The listing builds one solid part. Answer for the finished solid, in the listing's coordinates (mm). Face numbers are marked on the shaded views. A direction names the side the tool comes from. Round coordinates to 2 decimals unless told otherwise and drop trailing zeros. Write each loop counter-clockwise with the first axis right and the second up, starting at its lowest first coordinate (ties: lowest second). Pieces come first, ordered by that corner, then holes.
(1) For the marked faces 4 and 5, determine the directions among +Z, -Z, +X, -X, +Y, -Y from which every point of the face is accessible in a straight line to the end or side of a thin tool.
(2) The mould has two halves that part along Y. Classify the marked faces 1, 2 and 3: +Y half, -Y half, draft (parallel to the pull), parting line (faces both ways), or undercut.
(3) A cutting plane is placed at A-A, the plane z = 7.25. Give the vertices of the cut face in (x, y).
(4) Find the intervals of material crossed by probe 1 along Y at (x, z) = (80, 0.6); probe 2 along X at (y, z) = (37, 9.75); probe 3 along Y at (x, z) = (5, 1.75), in increasing order.
(5) A cutting plane is placed at C-C, the plane x = 31.5. Give the vertices of the cut face in (y, z), and give its area (3 significant figures).
(6) Each of these flat-tipped pins is pushed along its axis until it touches: pin 1 Ø0.8 at (x, z) = (13, 0.5) entering from -Y; pin 2 Ø1.1 at (x, y) = (79.5, 5.5) entering from +Z. Where does it stop, or does it pass through?
(7) A cutting plane is placed at B-B, the plane x = 10. Give the vertices of the cut face in (y, z).
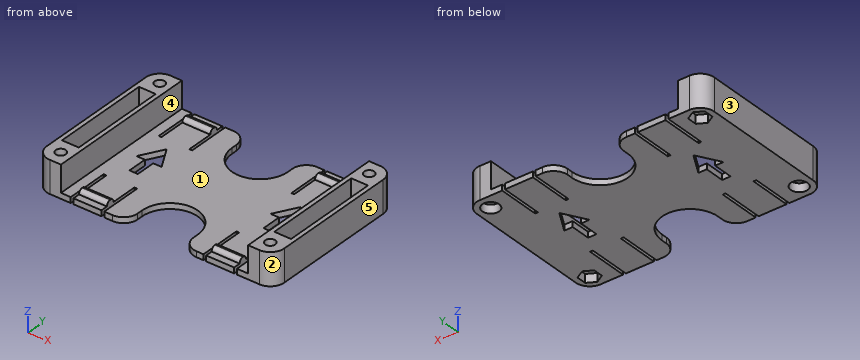
from build123d import *

# Parameters (mm, degrees)
PAD_DEPTH       = 11.5
SKETCH001_W     = 67
SKETCH001_H     = 65
POCKET_DEPTH    = 9.5
SKETCH002_R     = 3
POCKET001_DEPTH = 3
SKETCH003_W     = 6
SKETCH003_H     = 35
POCKET002_DEPTH = 9.5
SKETCH004_R     = 1.8
POCKET003_DEPTH = 8.3
SKETCH006_W     = 1
SKETCH006_H     = 15
POCKET004_DEPTH = 5
SKETCH007_W     = 1
SKETCH007_H     = 15
POCKET005_DEPTH = 5
SKETCH008_W     = 10
SKETCH008_H     = 3
PAD001_DEPTH    = 1.5
FILLET_R        = 1.4
POCKET006_DEPTH = 5


with BuildPart() as part:
    # Sketch → Pad (new body)
    with BuildSketch(Plane.XY):
        with BuildLine():
            ThreePointArc((0, 5), (1.464466, 1.464466), (5, 0))
            Line((5, 0), (27.5, 0))
            ThreePointArc((27.5, 0), (31.035534, 1.464466), (32.5, 5))
            Line((32.5, 5), (32.5, 7))
            ThreePointArc((52.5, 7), (42.5, 17), (32.5, 7))
            Line((52.5, 7), (52.5, 5))
            ThreePointArc((52.5, 5), (53.964466, 1.464466), (57.5, 0))
            Line((57.5, 0), (80, 0))
            ThreePointArc((80, 0), (83.535534, 1.464466), (85, 5))
            Line((85, 50), (85, 5))
            ThreePointArc((85, 50), (83.535534, 53.535534), (80, 55))
            Line((57.5, 55), (80, 55))
            ThreePointArc((57.5, 55), (53.964466, 53.535534), (52.5, 50))
            Line((52.5, 50), (52.5, 48))
            ThreePointArc((32.5, 48), (42.5, 38), (52.5, 48))
            Line((32.5, 50), (32.5, 48))
            ThreePointArc((32.5, 50), (31.035534, 53.535534), (27.5, 55))
            Line((5, 55), (27.5, 55))
            ThreePointArc((5, 55), (1.464466, 53.535534), (0, 50))
            Line((0, 5), (0, 50))
        make_face()
    extrude(amount=PAD_DEPTH)

    # Sketch001 → Pocket (cut)
    with BuildSketch(Plane.XY.offset(11.5)):
        with Locations((42.5, 27.5)):
            Rectangle(SKETCH001_W, SKETCH001_H)
    extrude(amount=-POCKET_DEPTH, mode=Mode.SUBTRACT)

    # Sketch002 → Pocket001 (cut)
    with BuildSketch(Plane(origin=(0, 0, 0), x_dir=(1, 0, 0), z_dir=(0, 0, -1))):
        with Locations((80, -50)):
            Circle(SKETCH002_R)
        with Locations((5, -5)):
            Circle(SKETCH002_R)
        Polygon((2, -51.732051), (2, -48.267949), (5, -46.535898), (8, -48.267949), (8, -51.732051), (5, -53.464102), align=None)
        Polygon((77, -3.267949), (77, -6.732051), (80, -8.464102), (83, -6.732051), (83, -3.267949), (80, -1.535898), align=None)
    extrude(amount=-POCKET001_DEPTH, mode=Mode.SUBTRACT)

    # Sketch003 → Pocket002 (cut)
    with BuildSketch(Plane.XY.offset(11.5)):
        with Locations((4.5, 27.5)):
            Rectangle(SKETCH003_W, SKETCH003_H)
        with Locations((80.5, 27.5)):
            Rectangle(SKETCH003_W, SKETCH003_H)
    extrude(amount=-POCKET002_DEPTH, mode=Mode.SUBTRACT)

    # Sketch004 → Pocket003 (cut)
    with BuildSketch(Plane.XY.offset(11.5)):
        with Locations((5, 50)):
            Circle(SKETCH004_R)
        with Locations((80, 50)):
            Circle(SKETCH004_R)
        with Locations((80, 5)):
            Circle(SKETCH004_R)
        with Locations((5, 5)):
            Circle(SKETCH004_R)
    extrude(amount=-POCKET003_DEPTH, mode=Mode.SUBTRACT)

    # Sketch006 → Pocket004 (cut)
    with BuildSketch(Plane.XY.offset(2)):
        with Locations((71.5, 47.5)):
            Rectangle(SKETCH006_W, SKETCH006_H)
        with Locations((60.5, 47.5)):
            Rectangle(SKETCH006_W, SKETCH006_H)
        with Locations((24, 47.5)):
            Rectangle(SKETCH006_W, SKETCH006_H)
        with Locations((13, 47.5)):
            Rectangle(SKETCH006_W, SKETCH006_H)
    extrude(amount=-POCKET004_DEPTH, mode=Mode.SUBTRACT)

    # Sketch007 → Pocket005 (cut)
    with BuildSketch(Plane.XY.offset(2)):
        with Locations((71.5, 7.5)):
            Rectangle(SKETCH007_W, SKETCH007_H)
        with Locations((60.5, 7.5)):
            Rectangle(SKETCH007_W, SKETCH007_H)
        with Locations((24, 7.5)):
            Rectangle(SKETCH007_W, SKETCH007_H)
        with Locations((13, 7.5)):
            Rectangle(SKETCH007_W, SKETCH007_H)
    extrude(amount=-POCKET005_DEPTH, mode=Mode.SUBTRACT)

    # Sketch008 → Pad001 (new body)
    with BuildSketch(Plane.XY.offset(2)):
        with Locations((18.5, 4)):
            Rectangle(SKETCH008_W, SKETCH008_H)
        with Locations((66, 4)):
            Rectangle(SKETCH008_W, SKETCH008_H)
        with Locations((18.5, 51)):
            Rectangle(SKETCH008_W, SKETCH008_H)
        with Locations((66, 51)):
            Rectangle(SKETCH008_W, SKETCH008_H)
    extrude(amount=PAD001_DEPTH)

    # Fillet
    fillet_edges = [part.edges().sort_by_distance(p)[0] for p in [
        (18.5, 49.5, 3.5),
        (18.5, 52.5, 3.5),
        (66, 52.5, 3.5),
        (66, 49.5, 3.5),
        (66, 5.5, 3.5),
        (66, 2.5, 3.5),
        (18.5, 2.5, 3.5),
        (18.5, 5.5, 3.5),
    ]]
    fillet(fillet_edges, radius=FILLET_R)

    # Sketch005 → Pocket006 (cut)
    with BuildSketch(Plane.XY.offset(2)):
        Polygon((17, 28), (14, 28), (18.5, 36), (23, 28), (20, 28), (20, 21), (17, 21), align=None)
        Polygon((65, 28), (62, 28), (66.5, 36), (71, 28), (68, 28), (68, 21), (65, 21), align=None)
    extrude(amount=-POCKET006_DEPTH, mode=Mode.SUBTRACT)


solid = part.part
Solutions:
1. face 4: +Z, +Y, -Y
1. face 5: +Z, -Z, +X, +Y, -Y
2. face 1: undercut
2. face 2: -Y half
2. face 3: draft
3. outline: (0, 5) arc R5 ccw to (5, 0) - (9, 0) - (9, 55) - (5, 55) arc R5 ccw to (0, 50) - close; (76, 0) - (80, 0) arc R5 ccw to (85, 5) - (85, 50) arc R5 ccw to (80, 55) - (76, 55) - close; hole (1.5, 10) - (7.5, 10) - (7.5, 45) - (1.5, 45) - close; hole circle Ø3.6 at (5, 5); hole circle Ø3.6 at (5, 50); hole (77.5, 10) - (83.5, 10) - (83.5, 45) - (77.5, 45) - close; hole circle Ø3.6 at (80, 5); hole circle Ø3.6 at (80, 50)
4. probe 1: y = 0 to 1.54, 8.46 to 47, 53 to 55
4. probe 2: x = 0 to 1.5, 7.5 to 9, 76 to 77.5, 83.5 to 85
4. probe 3: y = 0 to 2, 8 to 46.54, 53.46 to 55
5. outline: (2, 0) - (53, 0) - (53, 2) - (2, 2) - close
5. area: 102 mm2
6. pin 1: stops at y = 15
6. pin 2: stops at z = 3.2
7. outline: (0, 0) - (55, 0) - (55, 2) - (0, 2) - close
